Verification items for the finished model (mm, model axes). A direction names the side the tool comes from. Round coordinates to 2 decimals unless told otherwise and drop trailing zeros. Loops run counter-clockwise (first coordinate to the right, second up) from the corner with the lowest first, then second, coordinate; pieces in that order, holes last. Notation, with made-up numbers: (50, -20) -> (86, -20) arc R13 ccw to (86, -10) -> close; hole circle Ø4 at (40.5, 16.25). An arc over 180 degrees is marked (long way). Write item = value, one per line. Start each with the question number.
```python
from build123d import *

# Parameters (mm, degrees)
SKETCH1_W           = 115
SKETCH1_H           = 140
BOSS_EXTRUDE1_DEPTH = 2.4
CUT_EXTRUDE1_DEPTH  = 3.4
FILLET1_R           = 10
SKETCH3_W           = 2.4
SKETCH3_H           = 140
BOSS_EXTRUDE2_DEPTH = 25
FILLET2_R           = 10
SKETCH4_R           = 2.75
CUT_EXTRUDE2_DEPTH  = 116
SKETCH5_R           = 14.275
CUT_EXTRUDE3_DEPTH  = 3.4


with BuildPart() as part:
    # Sketch1 → Boss-Extrude1 (new body)
    with BuildSketch(Plane(origin=(0, 0, 0), x_dir=(0, 0, -1), z_dir=(1, 0, 0))):
        with Locations((57.5, -70)):
            Rectangle(SKETCH1_W, SKETCH1_H)
    extrude(amount=BOSS_EXTRUDE1_DEPTH)

    # Sketch2 → Cut-Extrude1 (cut, through all)
    with BuildSketch(Plane(origin=(2.4, 0, 0), x_dir=(0, 0, -1), z_dir=(1, 0, 0))):
        Polygon((87, 0), (115, -30), (142.616199658, -32.505405645), (142.616199658, 14.875556406), align=None)
        Polygon((115, -110), (87, -140), (87, -152.661109726), (136.310004643, -152.661109726), align=None)
    extrude(amount=-CUT_EXTRUDE1_DEPTH, mode=Mode.SUBTRACT)

    # Fillet1
    fillet1_edges = [part.edges().sort_by_distance(p)[0] for p in [
        (1.2, 0, -87),
        (1.2, -30, -115),
        (1.2, -110, -115),
        (1.2, -140, -87),
    ]]
    fillet(fillet1_edges, radius=FILLET1_R)

    # Sketch3 → Boss-Extrude2 (add)
    with BuildSketch(Plane(origin=(2.4, 0, 0), x_dir=(0, 0, -1), z_dir=(1, 0, 0))):
        with Locations((1.2, -70)):
            Rectangle(SKETCH3_W, SKETCH3_H)
    extrude(amount=BOSS_EXTRUDE2_DEPTH)

    # Fillet2
    fillet2_edges = [part.edges().sort_by_distance(p)[0] for p in [
        (27.4, -140, -1.2),
        (27.4, 0, -1.2),
    ]]
    fillet(fillet2_edges, radius=FILLET2_R)

    # Sketch4 → Cut-Extrude2 (cut, through all)
    with BuildSketch(Plane.XY):
        with Locations((11.974983581, -70)):
            Circle(SKETCH4_R)
        with Locations((11.974983581, -25)):
            Circle(SKETCH4_R)
        with Locations((11.974983581, -115)):
            Circle(SKETCH4_R)
    extrude(amount=-CUT_EXTRUDE2_DEPTH, mode=Mode.SUBTRACT)

    # Sketch5 → Cut-Extrude3 (cut, through all)
    with BuildSketch(Plane(origin=(2.4, 0, 0), x_dir=(0, 0, -1), z_dir=(1, 0, 0))):
        with Locations((22.591699334, -20)):
            Circle(SKETCH5_R)
    extrude(amount=-CUT_EXTRUDE3_DEPTH, mode=Mode.SUBTRACT)


solid = part.part
```
(1) Section check A-A on y = -25. Enter the section's corners in (x, z).
(2) Scan lines: line 1 (Z direction, x = 8.5, y = -64); line 2 (X direction, y = -122, z = -67.5). Record each from-to range of solid material in increasing order. Write a range as [from, to].
(3) Access from +Z, -Z, +X, -X, +Y, -Y to the whole of each face (thin tool, end or side, straight path). Record for faces 1 (the flat face through (17, -71, 0)), 2 (the flat face through (15, -71, -2.4)).
(4) Depth check by flat-ended pin: pin 1 Ø1 at (x, y) = (11.5, -110) entering from +Z; pin 2 Ø12 at (x, y) = (23, -45) entering from -Z; pin 3 Ø2 at (y, z) = (-51, -102) entering from +X; pin 4 Ø1.5 at (x, z) = (4.5, -85.5) entering from -Y. Enter the tip coordinate at first touch or a pass-through.
(5) Draft check along X on faces 3 (the cylindrical face through (24.39, -137.15, -1.22)), 4 (the cylindrical face through (11.617, -67.273, -1.183)), 5 (the flat face through (2, 0, -35)). Enter one of: +X half, -X half, draft (parallel to the pull), parting line (faces both ways), or undercut.
(6) Section check D-D on y = -115. Enter the section's corners in (x, z), then the cut area to 3 significant figures.
(7) Section check C-C on z = -17. Enter the section's corners in (x, y), then the cut area to 3 significant figures.
(8) Section check B-B on x = 13. Enter the section's corners in (y, z), then the cut area to 3 significant figures.
Computed values:
q1.outline = (0, -110.33) -> (2.4, -110.33) -> (2.4, -35.96) -> (0, -35.96) -> close; (0, -9.22) -> (2.4, -9.22) -> (2.4, -2.4) -> (9.22, -2.4) -> (9.22, 0) -> (0, 0) -> close; (14.72, -2.4) -> (27.4, -2.4) -> (27.4, 0) -> (14.72, 0) -> close
q2.line_1 = [-2.4, 0]
q2.line_2 = [0, 2.4]
q3.face_1 = +Z, +X, -X, +Y, -Y
q3.face_2 = -Z, +X, +Y, -Y
q4.pin_1 = 0
q4.pin_2 = -2.4
q4.pin_3 = 2.4
q4.pin_4 = through
q5.face_3 = +X half
q5.face_4 = undercut
q5.face_5 = draft
q6.outline = (0, -110.33) -> (2.4, -110.33) -> (2.4, -2.4) -> (9.22, -2.4) -> (9.22, 0) -> (0, 0) -> close; (14.72, -2.4) -> (27.4, -2.4) -> (27.4, 0) -> (14.72, 0) -> close
q6.area = 312 mm²
q7.outline = (0, -140) -> (2.4, -140) -> (2.4, -33.13) -> (0, -33.13) -> close; (0, -6.87) -> (2.4, -6.87) -> (2.4, 0) -> (0, 0) -> close
q7.area = 273 mm²
q8.outline = (-140, -2.4) -> (-117.55, -2.4) -> (-117.55, 0) -> (-140, 0) -> close; (-112.45, -2.4) -> (-72.55, -2.4) -> (-72.55, 0) -> (-112.45, 0) -> close; (-67.45, -2.4) -> (-27.55, -2.4) -> (-27.55, 0) -> (-67.45, 0) -> close; (-22.45, -2.4) -> (0, -2.4) -> (0, 0) -> (-22.45, 0) -> close
q8.area = 299 mm²
